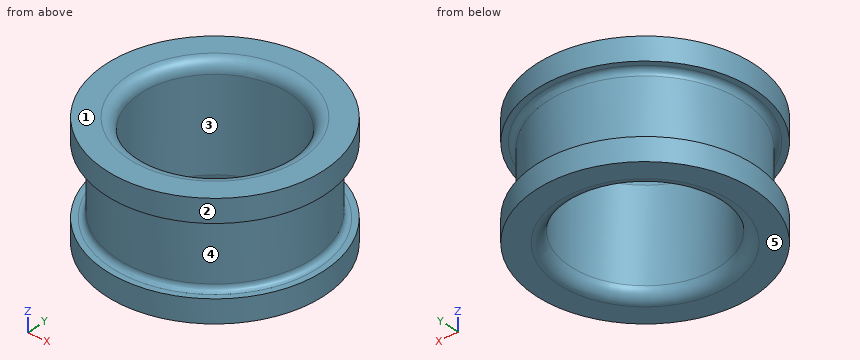
from build123d import *

# Parameters (mm, degrees)
SKETCH1_R               = 9.5
BOSS_EXTRUDE1_DEPTH     = 2
SKETCH2_R               = 8.5
BOSS_EXTRUDE2_DEPTH     = 6
SKETCH3_R               = 9.5
BOSS_EXTRUDE3_DEPTH     = 2
CUT_EXTRUDE1_DEPTH      = 17.748134224
CUT_EXTRUDE1_DEPTH_BACK = 17.748134224
SKETCH4_R               = 6.5
FILLET1_R               = 1
FILLET2_R               = 0.5


with BuildPart() as part:
    # Sketch1 → Boss-Extrude1 (new body)
    with BuildSketch(Plane.XY):
        Circle(SKETCH1_R)
    extrude(amount=BOSS_EXTRUDE1_DEPTH)

    # Sketch2 → Boss-Extrude2 (add)
    with BuildSketch(Plane.XY.offset(2)):
        Circle(SKETCH2_R)
    extrude(amount=BOSS_EXTRUDE2_DEPTH)

    # Sketch3 → Boss-Extrude3 (add)
    with BuildSketch(Plane.XY.offset(8)):
        Circle(SKETCH3_R)
    extrude(amount=BOSS_EXTRUDE3_DEPTH)

    # Sketch4 → Cut-Extrude1 (cut, two sides: drawn at the far end of the back side and taken through both)
    with BuildSketch(Plane(origin=(0, 0, 0), x_dir=(-1, 0, 0), z_dir=(0, 0, -1)).offset(-CUT_EXTRUDE1_DEPTH_BACK)):
        Circle(SKETCH4_R)
    extrude(amount=CUT_EXTRUDE1_DEPTH + CUT_EXTRUDE1_DEPTH_BACK, mode=Mode.SUBTRACT)

    # Fillet1
    fillet1_edges = [part.edges().sort_by_distance(p)[0] for p in [
        (6.5, 0, 10),
        (6.5, 0, 0),
    ]]
    fillet(fillet1_edges, radius=FILLET1_R)

    # Fillet2
    fillet2_edges = [part.edges().sort_by_distance(p)[0] for p in [
        (-8.5, 0, 2),
        (-8.5, 0, 8),
    ]]
    fillet(fillet2_edges, radius=FILLET2_R)


solid = part.part
For this review, take the finished solid that the model builds, in its own axes (mm). Face numbers are marked on the shaded views. A direction names the side the tool comes from. Coordinates: 2 decimals unless noted, no trailing zeros. Loops run counter-clockwise (first coordinate to the right, second up) from the corner with the lowest first, then second, coordinate; pieces in that order, holes last. Notation, with made-up numbers: (30.5, 49.25) - (37.5, 49.25) arc R22 cw to (37.5, 69.25) - close; hole circle Ø10 at (18.25, -31). An arc over 180 degrees is marked (long way). Use a Markdown table: item, result. Add a question column.
Item 1: Insertion check: pin 1 Ø2 at (x, z) = (4.5, 2.5) entering from +Y; pin 2 Ø2 at (x, y) = (3.5, 2.5) entering from +Z. Each pin has a flat end and moves straight along its axis. Give the tip position at first contact, or say it passes through.
Item 2: For line 1 (Y direction, x = 0, z = 6.5); line 2 (Z direction, x = -7, y = -2.5); line 3 (Z direction, x = 6.75, y = 6), list the stretches that pass through material, from the lowest coordinate up.
Item 3: We need section C-C (z = 4.5). Give the boundary of the cut face in (x, y).
Item 4: Mouldability with a two-part tool opening along X and no side actions: class the marked faces 1, 2 and 3 as pulls with the +X half, pulls with the -X half, needs draft (parallel to the pull), parting line crosses it, or undercut.
Item 5: We need section A-A (y = 0). Give the boundary of the cut face in (x, z), and give its area (3 significant figures).
Item 6: We need section D-D (z = 2.25). Give the boundary of the cut face in (x, y), and give its area (3 significant figures).
Item 7: Tool access review of the marked faces 4 and 5: name each direction out of +Z, -Z, +X, -X, +Y, -Y from which nothing blocks a thin tool from reaching the whole face with its end or side.
Results list:
| question | item | result |
|---|---|---|
| 1 | pin 1 | stops at y = 8.78 |
| 1 | pin 2 | passes through |
| 2 | line 1 | y = -8.5 to -6.5, 6.5 to 8.5 |
| 2 | line 2 | z = 0 to 10 |
| 2 | line 3 | z = 0 to 2, 8 to 10 |
| 3 | outline | circle Ø17 at (0, 0); hole circle Ø13 at (0, 0) |
| 4 | face 1 | needs draft |
| 4 | face 2 | parting line crosses it |
| 4 | face 3 | undercut |
| 5 | outline | (-9.5, 0) - (-7.5, 0) arc R1 ccw to (-6.5, 1) - (-6.5, 9) arc R1 ccw to (-7.5, 10) - (-9.5, 10) - (-9.5, 8) - (-9, 8) arc R0.5 cw to (-8.5, 7.5) - (-8.5, 2.5) arc R0.5 cw to (-9, 2) - (-9.5, 2) - close; (6.5, 1) arc R1 ccw to (7.5, 0) - (9.5, 0) - (9.5, 2) - (9, 2) arc R0.5 cw to (8.5, 2.5) - (8.5, 7.5) arc R0.5 cw to (9, 8) - (9.5, 8) - (9.5, 10) - (7.5, 10) arc R1 ccw to (6.5, 9) - close |
| 5 | area | 47.4 mm^2 |
| 6 | outline | circle Ø17.13 at (0, 0); hole circle Ø13 at (0, 0) |
| 6 | area | 97.8 mm^2 |
| 7 | face 4 | none |
| 7 | face 5 | -Z, +X, -X, +Y, -Y |
